Could you check a few things on this model? Use its own coordinates, in mm. Give positions to 0.01 mm unless a question says otherwise; leave off trailing zeros. Order: outer loops, then holes, each group sorted by start corner. A loop starts at its lowest first (then second) coordinate and runs counter-clockwise, first axis right, second up.
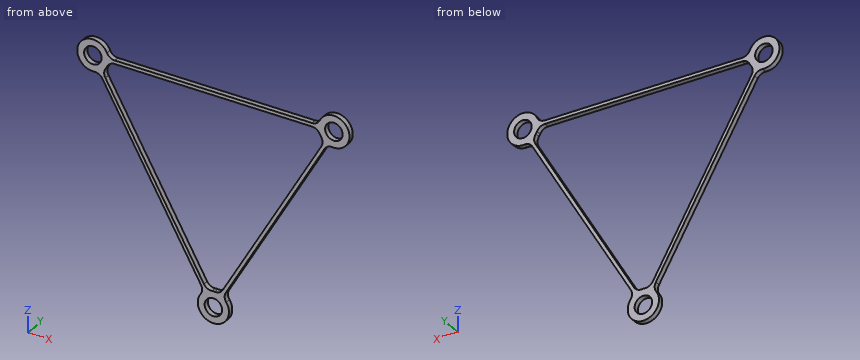
from build123d import *

# Parameters (mm, degrees)
SKETCH2_R        = 2.55
MAIN_SHAPE_DEPTH = 0.75
OUTSIDE_FILLET_R = 2.5
INSIDE_FILLET_R  = 2.5


with BuildPart() as part:
    # Sketch2 → main_shape (new body, symmetric)
    with BuildSketch(Plane(origin=(0, 0, 0), x_dir=(1, 0, 0), z_dir=(0, 1, 0))):
        with BuildLine():
            Line((-33.271790687, -16.098443032), (-2.694234717, 36.86343748))
            ThreePointArc((-2.694234717, 36.86343748), (0, 45.079988897), (2.694234717, 36.86343748))
            Line((2.694234717, 36.86343748), (33.271790687, -16.098443032))
            ThreePointArc((33.271790687, -16.098443032), (39.040415587, -22.539994449), (30.57755597, -20.764994449))
            Line((30.57755597, -20.764994449), (-30.57755597, -20.764994449))
            ThreePointArc((-30.57755597, -20.764994449), (-39.040415587, -22.539994449), (-33.271790687, -16.098443032))
        make_face()
        with Locations((0, 40.529988897)):
            Circle(SKETCH2_R, mode=Mode.SUBTRACT)
        with Locations((35.1, -20.264994449)):
            Circle(SKETCH2_R, mode=Mode.SUBTRACT)
        with Locations((-35.1, -20.264994449)):
            Circle(SKETCH2_R, mode=Mode.SUBTRACT)
        with BuildLine():
            Line((-30.57755597, -19.764994449), (30.57755597, -19.764994449))
            ThreePointArc((30.57755597, -19.764994449), (31.159584413, -17.989994449), (32.405765283, -16.598443032))
            Line((32.405765283, -16.598443032), (1.828209313, 36.36343748))
            ThreePointArc((1.828209313, 36.36343748), (0, 35.979988897), (-1.828209313, 36.36343748))
            Line((-1.828209313, 36.36343748), (-32.405765283, -16.598443032))
            ThreePointArc((-32.405765283, -16.598443032), (-31.159584413, -17.989994449), (-30.57755597, -19.764994449))
        make_face(mode=Mode.SUBTRACT)
    extrude(amount=MAIN_SHAPE_DEPTH, both=True)

    # outside_fillet
    outside_fillet_edges = [part.edges().sort_by_distance(p)[0] for p in [
        (-33.271790687, 0, 16.098443032),
        (-2.694234717, 0, -36.86343748),
        (2.694234717, 0, -36.86343748),
        (33.271790687, 0, 16.098443032),
        (30.57755597, 0, 20.764994449),
        (-30.57755597, 0, 20.764994449),
    ]]
    fillet(outside_fillet_edges, radius=OUTSIDE_FILLET_R)

    # inside_fillet
    inside_fillet_edges = [part.edges().sort_by_distance(p)[0] for p in [
        (1.828209313, 0, -36.36343748),
        (-1.828209313, 0, -36.36343748),
        (-32.405765283, 0, 16.598443032),
        (-30.57755597, 0, 19.764994449),
        (30.57755597, 0, 19.764994449),
        (32.405765283, 0, 16.598443032),
    ]]
    fillet(inside_fillet_edges, radius=INSIDE_FILLET_R)


solid = part.part
Item 1: Please list where these lines run through material, in increasing order: line 1 along X through (y, z) = (-0.35, 16.5); line 2 along Z through (x, y) = (35.1, 0.25) (3 decimals); line 3 along X through (y, z) = (0.5, -40).
Findings:
line 1: x = -37.65 to -31.8, 31.8 to 37.65
line 2: z = 15.715 to 17.715, 22.815 to 24.815
line 3: x = -4.52 to -2.49, 2.49 to 4.52
Item 2: Imagine slicing it at B-B on x = 17. List the corners of the cut face in (y, z) for me (3 decimals).
Findings:
outline: (-0.75, -12.085) - (0.75, -12.085) - (0.75, -10.085) - (-0.75, -10.085) - close; (-0.75, 19.765) - (0.75, 19.765) - (0.75, 20.765) - (-0.75, 20.765) - close
Item 3: For pin 1 (8 mm diameter, centred on x = 0, z = -40.53, fed in from -Y), with a flat end and sliding along its axis, tell me the tip position at first contact or that it passes through.
Findings:
pin 1: stops at y = -0.75
Item 4: Imagine slicing it at C-C on y = -0.2. Give the number of separate pieces and of enclosed holes in the cut face, then the cut area to 3 significant figures.
Findings:
separate pieces: 1
enclosed holes: 4
area: 324 mm2
Item 5: Imagine slicing it at A-A on z = -16. List the corners of the cut face in (x, y) for me.
Findings:
outline: (-14.74, -0.75) - (-13.59, -0.75) - (-13.59, 0.75) - (-14.74, 0.75) - close; (13.59, -0.75) - (14.74, -0.75) - (14.74, 0.75) - (13.59, 0.75) - close
